For this review, use the dimensioned drawing (mm, ordinates from the lowest corner) and the shaded views. Round coordinates to 2 decimals unless told otherwise and drop trailing zeros. Write each loop counter-clockwise with the first axis right and the second up, starting at its lowest first coordinate (ties: lowest second). Pieces come first, ordered by that corner, then holes. Notation, with made-up numbers: M 56.25,-36 L 96.25,-36 A22 ccw 96.25,-30 Z; hole C 21.5,-4.75 d8. An arc over 180 degrees is marked long. Use CSV: the item, a comma, the result in double quotes.
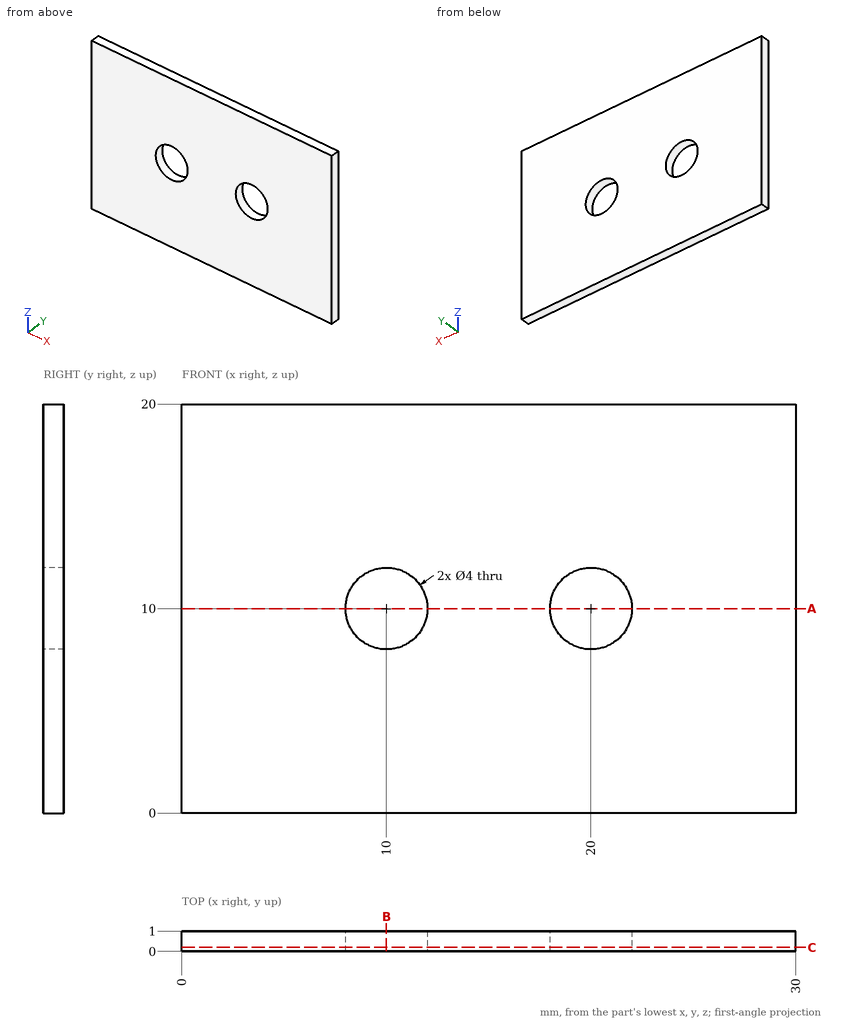
1) Wall thickness on line 1 along X through (y, z) = (0.6, 9.5); line 2 along Z through (x, y) = (10, 0.45); line 3 along X through (y, z) = (0.75, 9.75): over which ranges is each line inside the solid? List them lowest first. Write a range as [from, to].
Answers:
line 1,"[0, 8.06], [11.94, 18.06], [21.94, 30]"
line 2,"[0, 8], [12, 20]"
line 3,"[0, 8.02], [11.98, 18.02], [21.98, 30]"
2) Add section B-B on x = 10. Write out the cut boundary in (y, z), then the cut area to 3 significant figures.
Answers:
outline,"M 0,0 L 1,0 L 1,8 L 0,8 Z; M 0,12 L 1,12 L 1,20 L 0,20 Z"
area,"16.0 mm²"
3) Add section A-A on z = 10. Write out the cut boundary in (x, y), then the cut area to 3 significant figures.
Answers:
outline,"M 0,0 L 8,0 L 8,1 L 0,1 Z; M 12,0 L 18,0 L 18,1 L 12,1 Z; M 22,0 L 30,0 L 30,1 L 22,1 Z"
area,"22.0 mm²"
4) Add section C-C on y = 0.2. Write out the cut boundary in (x, z), then the cut area to 3 significant figures.
Answers:
outline,"M 0,0 L 30,0 L 30,20 L 0,20 Z; hole C 10,10 d4; hole C 20,10 d4"
area,"575 mm²"
